```python
from build123d import *

# Parameters (mm, degrees)
BOSS_EXTRUDE1_START  = -85
SKETCH1_W            = 80
SKETCH1_H            = 34
BOSS_EXTRUDE1_DEPTH  = 170
BOSS_EXTRUDE2_START  = -83
SKETCH2_W            = 76
SKETCH2_H            = 38
BOSS_EXTRUDE2_DEPTH  = 166
BOSS_EXTRUDE3_START  = -45
SKETCH3_W            = 23.6
SKETCH3_H            = 12.6
BOSS_EXTRUDE3_DEPTH  = 90
BOSS_EXTRUDE4_START  = -45
SKETCH4_R            = 0.9
BOSS_EXTRUDE4_DEPTH  = 90
BOSS_EXTRUDE5_START  = -45
SKETCH5_R            = 0.9
BOSS_EXTRUDE5_DEPTH  = 90
BOSS_EXTRUDE6_START  = -45
SKETCH6_W            = 23.6
SKETCH6_H            = 12.6
BOSS_EXTRUDE6_DEPTH  = 90
BOSS_EXTRUDE7_START  = -45
SKETCH7_R            = 0.9
BOSS_EXTRUDE7_DEPTH  = 90
BOSS_EXTRUDE8_START  = -45
SKETCH8_R            = 0.9
BOSS_EXTRUDE8_DEPTH  = 90
BOSS_EXTRUDE9_START  = -45
SKETCH9_W            = 10
SKETCH9_H            = 6
BOSS_EXTRUDE9_DEPTH  = 90
BOSS_EXTRUDE10_START = -90
SKETCH10_W           = 10
SKETCH10_H           = 6
BOSS_EXTRUDE10_DEPTH = 10
BOSS_EXTRUDE11_START = -90
SKETCH11_W           = 10
SKETCH11_H           = 5
BOSS_EXTRUDE11_DEPTH = 10
BOSS_EXTRUDE12_START = -90
SKETCH12_W           = 19
SKETCH12_H           = 13
BOSS_EXTRUDE12_DEPTH = 10
BOSS_EXTRUDE13_START = 62
SKETCH13_W           = 12
SKETCH13_H           = 4
BOSS_EXTRUDE13_DEPTH = 10
BOSS_EXTRUDE14_START = 62
SKETCH14_W           = 12
SKETCH14_H           = 4
BOSS_EXTRUDE14_DEPTH = 10
BOSS_EXTRUDE15_START = -80
SKETCH15_W           = 12
SKETCH15_H           = 4
BOSS_EXTRUDE15_DEPTH = 10
BOSS_EXTRUDE16_START = -45
SKETCH16_R           = 0.9
BOSS_EXTRUDE16_DEPTH = 90
BOSS_EXTRUDE17_START = -45
SKETCH17_R           = 0.9
BOSS_EXTRUDE17_DEPTH = 90


with BuildPart() as part:
    # Sketch1 → Boss-Extrude1 (new body)
    with BuildSketch(Plane.XY.offset(BOSS_EXTRUDE1_START)):
        with Locations((0, 17)):
            Rectangle(SKETCH1_W, SKETCH1_H)
    extrude(amount=BOSS_EXTRUDE1_DEPTH)


with BuildPart() as body_2:
    # Sketch2 → Boss-Extrude2 (new body)
    with BuildSketch(Plane.XY.offset(BOSS_EXTRUDE2_START)):
        with Locations((0, 21)):
            Rectangle(SKETCH2_W, SKETCH2_H)
    extrude(amount=BOSS_EXTRUDE2_DEPTH)


with BuildPart() as part_1:
    add(part.part)

    # Combine1: cut body 2
    add(body_2.part, mode=Mode.SUBTRACT)


with BuildPart() as body_2_2:
    # Sketch3 → Boss-Extrude3 (new body)
    with BuildSketch(Plane(origin=(0, 0, 0), x_dir=(0, 0, -1), z_dir=(1, 0, 0)).offset(BOSS_EXTRUDE3_START)):
        with Locations((-48.3, 19)):
            Rectangle(SKETCH3_W, SKETCH3_H)
    extrude(amount=BOSS_EXTRUDE3_DEPTH)


with BuildPart() as part_2:
    add(part_1.part)

    # Combine2: cut body 2 2
    add(body_2_2.part, mode=Mode.SUBTRACT)


with BuildPart() as body_2_3:
    # Sketch4 → Boss-Extrude4 (new body)
    with BuildSketch(Plane(origin=(0, 0, 0), x_dir=(0, 0, -1), z_dir=(1, 0, 0)).offset(BOSS_EXTRUDE4_START)):
        with Locations(Location((-34.3, 19, 0), (0, 0, 180))):
            Circle(SKETCH4_R)
    extrude(amount=BOSS_EXTRUDE4_DEPTH)


with BuildPart() as part_3:
    add(part_2.part)

    # Combine3: cut body 2 3
    add(body_2_3.part, mode=Mode.SUBTRACT)


with BuildPart() as body_2_4:
    # Sketch5 → Boss-Extrude5 (new body)
    with BuildSketch(Plane(origin=(0, 0, 0), x_dir=(0, 0, -1), z_dir=(1, 0, 0)).offset(BOSS_EXTRUDE5_START)):
        with Locations(Location((-62.3, 19, 0), (0, 0, 180))):
            Circle(SKETCH5_R)
    extrude(amount=BOSS_EXTRUDE5_DEPTH)


with BuildPart() as part_4:
    add(part_3.part)

    # Combine4: cut body 2 4
    add(body_2_4.part, mode=Mode.SUBTRACT)


with BuildPart() as body_2_5:
    # Sketch6 → Boss-Extrude6 (new body)
    with BuildSketch(Plane(origin=(0, 0, 0), x_dir=(0, 0, -1), z_dir=(1, 0, 0)).offset(BOSS_EXTRUDE6_START)):
        with Locations((62.3, 19)):
            Rectangle(SKETCH6_W, SKETCH6_H)
    extrude(amount=BOSS_EXTRUDE6_DEPTH)


with BuildPart() as part_5:
    add(part_4.part)

    # Combine5: cut body 2 5
    add(body_2_5.part, mode=Mode.SUBTRACT)


with BuildPart() as body_2_6:
    # Sketch7 → Boss-Extrude7 (new body)
    with BuildSketch(Plane(origin=(0, 0, 0), x_dir=(0, 0, -1), z_dir=(1, 0, 0)).offset(BOSS_EXTRUDE7_START)):
        with Locations(Location((76.3, 19, 0), (0, 0, 180))):
            Circle(SKETCH7_R)
    extrude(amount=BOSS_EXTRUDE7_DEPTH)


with BuildPart() as part_6:
    add(part_5.part)

    # Combine6: cut body 2 6
    add(body_2_6.part, mode=Mode.SUBTRACT)


with BuildPart() as body_2_7:
    # Sketch8 → Boss-Extrude8 (new body)
    with BuildSketch(Plane(origin=(0, 0, 0), x_dir=(0, 0, -1), z_dir=(1, 0, 0)).offset(BOSS_EXTRUDE8_START)):
        with Locations(Location((48.3, 19, 0), (0, 0, 180))):
            Circle(SKETCH8_R)
    extrude(amount=BOSS_EXTRUDE8_DEPTH)


with BuildPart() as part_7:
    add(part_6.part)

    # Combine7: cut body 2 7
    add(body_2_7.part, mode=Mode.SUBTRACT)


with BuildPart() as body_2_8:
    # Sketch9 → Boss-Extrude9 (new body)
    with BuildSketch(Plane(origin=(0, 0, 0), x_dir=(0, 0, -1), z_dir=(1, 0, 0)).offset(BOSS_EXTRUDE9_START)):
        with Locations((6, 24)):
            Rectangle(SKETCH9_W, SKETCH9_H)
    extrude(amount=BOSS_EXTRUDE9_DEPTH)


with BuildPart() as part_8:
    add(part_7.part)

    # Combine8: cut body 2 8
    add(body_2_8.part, mode=Mode.SUBTRACT)


with BuildPart() as body_2_9:
    # Sketch10 → Boss-Extrude10 (new body)
    with BuildSketch(Plane.XY.offset(BOSS_EXTRUDE10_START)):
        with Locations((0, 11)):
            Rectangle(SKETCH10_W, SKETCH10_H)
    extrude(amount=BOSS_EXTRUDE10_DEPTH)


with BuildPart() as part_9:
    add(part_8.part)

    # Combine9: cut body 2 9
    add(body_2_9.part, mode=Mode.SUBTRACT)


with BuildPart() as body_2_10:
    # Sketch11 → Boss-Extrude11 (new body)
    with BuildSketch(Plane.XY.offset(BOSS_EXTRUDE11_START)):
        with Locations((23, 8.5)):
            Rectangle(SKETCH11_W, SKETCH11_H)
    extrude(amount=BOSS_EXTRUDE11_DEPTH)


with BuildPart() as part_10:
    add(part_9.part)

    # Combine10: cut body 2 10
    add(body_2_10.part, mode=Mode.SUBTRACT)


with BuildPart() as body_2_11:
    # Sketch12 → Boss-Extrude12 (new body)
    with BuildSketch(Plane.XY.offset(BOSS_EXTRUDE12_START)):
        with Locations((-23.5, 15.5)):
            Rectangle(SKETCH12_W, SKETCH12_H)
    extrude(amount=BOSS_EXTRUDE12_DEPTH)


with BuildPart() as part_11:
    add(part_10.part)

    # Combine11: cut body 2 11
    add(body_2_11.part, mode=Mode.SUBTRACT)


with BuildPart() as body_2_12:
    # Sketch13 → Boss-Extrude13 (new body)
    with BuildSketch(Plane.XY.offset(BOSS_EXTRUDE13_START)):
        with Locations((-30, 1)):
            Rectangle(SKETCH13_W, SKETCH13_H)
    extrude(amount=BOSS_EXTRUDE13_DEPTH)


with BuildPart() as part_12:
    add(part_11.part)

    # Combine12: cut body 2 12
    add(body_2_12.part, mode=Mode.SUBTRACT)


with BuildPart() as body_2_13:
    # Sketch14 → Boss-Extrude14 (new body)
    with BuildSketch(Plane.XY.offset(BOSS_EXTRUDE14_START)):
        with Locations((30, 1)):
            Rectangle(SKETCH14_W, SKETCH14_H)
    extrude(amount=BOSS_EXTRUDE14_DEPTH)


with BuildPart() as part_13:
    add(part_12.part)

    # Combine13: cut body 2 13
    add(body_2_13.part, mode=Mode.SUBTRACT)


with BuildPart() as body_2_14:
    # Sketch15 → Boss-Extrude15 (new body)
    with BuildSketch(Plane.XY.offset(BOSS_EXTRUDE15_START)):
        with Locations((-24, 1)):
            Rectangle(SKETCH15_W, SKETCH15_H)
    extrude(amount=BOSS_EXTRUDE15_DEPTH)


with BuildPart() as part_14:
    add(part_13.part)

    # Combine14: cut body 2 14
    add(body_2_14.part, mode=Mode.SUBTRACT)


with BuildPart() as body_2_15:
    # Sketch16 → Boss-Extrude16 (new body)
    with BuildSketch(Plane(origin=(0, 0, 0), x_dir=(0, 0, -1), z_dir=(1, 0, 0)).offset(BOSS_EXTRUDE16_START)):
        with Locations(Location((30, 30, 0), (0, 0, 180))):
            Circle(SKETCH16_R)
    extrude(amount=BOSS_EXTRUDE16_DEPTH)


with BuildPart() as part_15:
    add(part_14.part)

    # Combine15: cut body 2 15
    add(body_2_15.part, mode=Mode.SUBTRACT)


with BuildPart() as body_2_16:
    # Sketch17 → Boss-Extrude17 (new body)
    with BuildSketch(Plane(origin=(0, 0, 0), x_dir=(0, 0, -1), z_dir=(1, 0, 0)).offset(BOSS_EXTRUDE17_START)):
        with Locations(Location((-30, 30, 0), (0, 0, 180))):
            Circle(SKETCH17_R)
    extrude(amount=BOSS_EXTRUDE17_DEPTH)


with BuildPart() as part_16:
    add(part_15.part)

    # Combine16: cut body 2 16
    add(body_2_16.part, mode=Mode.SUBTRACT)


solid = part_16.part
```
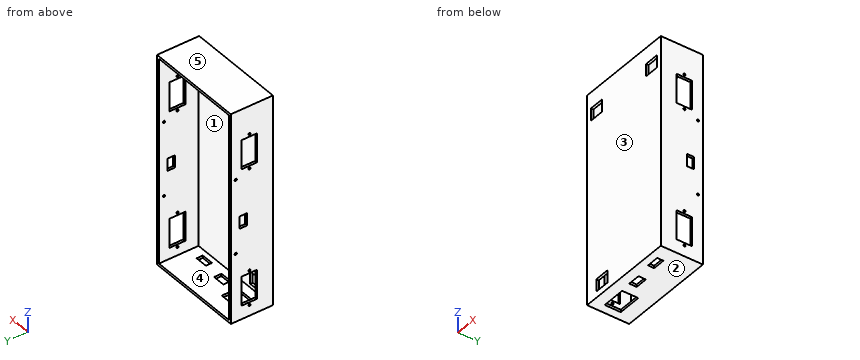
Here's how the part is built. I have some questions about the finished solid (model axes, mm). Face numbers are marked on the shaded views. A direction names the side the tool comes from. Give positions to 0.01 mm unless a question says otherwise; leave off trailing zeros. Order: outer loops, then holes, each group sorted by start corner. A loop starts at its lowest first (then second) coordinate and runs counter-clockwise, first axis right, second up. Notation, with made-up numbers: M 38.25,-27 L 84.25,-27 A19 ccw 84.25,9 Z; hole C 0.5,31 d11. An arc over 180 degrees is marked long. Use a Markdown table: item, result. Add a question column.
1. I need wall thicknesses on probe 1 along Y at (x, z) = (39.35, 30); probe 2 along Z at (x, y) = (-25, 5); probe 3 along X at (y, z) = (10.5, -61). Which ranges of each line are inside material? Lowest first, please. Write a range as from..to.
2. Suppose I cut it at B-B (z = 50). List the corners of the cut face in (x, y) for me.
3. Suppose I cut it at C-C (x = 12). List the corners of the cut face in (y, z) for me.
4. For pin 1 Ø6 at (x, z) = (-29.5, -46.5) entering from +Y, with a flat end and sliding along its axis, tell me the tip position at first contact or that it passes through.
5. If we mould it in two halves opening along Z, with no side actions, what happens to the marked faces 3, 4 and 5? For each: +Z half, -Z half, draft (parallel to the pull), parting line (faces both ways), or undercut.
6. On a 3-axis mill with a long thin cutter (end or side, diameter ignored), from which of +Z, -Z, +X, -X, +Y, -Y can I reach the whole of each face in a straight line? I mean the marked faces 1 and 2. Say none if no direction works.
7. Suppose I cut it at A-A (x = 0.5). List the corners of the cut face in (y, z) for me, and give its area (3 significant figures).
Results list:
| question | item | result |
|---|---|---|
| 1 | probe 1 | y = 0..29.1, 30.9..34 |
| 1 | probe 2 | z = -85..-83, 83..85 |
| 1 | probe 3 | x = -40..-38, 38..40 |
| 2 | outline | M -40,0 L 40,0 L 40,12.7 L 38,12.7 L 38,2 L -38,2 L -38,12.7 L -40,12.7 Z; M -40,25.3 L -38,25.3 L -38,34 L -40,34 Z; M 38,25.3 L 40,25.3 L 40,34 L 38,34 Z |
| 3 | outline | M 0,-85 L 34,-85 L 34,-83 L 2,-83 L 2,83 L 34,83 L 34,85 L 0,85 Z |
| 4 | pin 1 | stops at y = 2 |
| 5 | face 3 | draft |
| 5 | face 4 | undercut |
| 5 | face 5 | +Z half |
| 6 | face 1 | +Y |
| 6 | face 2 | -Z, +X, -X, +Y, -Y |
| 7 | outline | M 0,-85 L 8,-85 L 8,-83 L 2,-83 L 2,83 L 34,83 L 34,85 L 0,85 Z; M 14,-85 L 34,-85 L 34,-83 L 14,-83 Z |
| 7 | area | 456 mm² |
